Read the model definition and answer for the solid it produces. Units are mm, in the model's axes. Face numbers are marked on the shaded views. Give positions to 0.01 mm unless a question says otherwise; leave off trailing zeros. Write each loop counter-clockwise with the first axis right and the second up, starting at its lowest first coordinate (ties: lowest second). Pieces come first, ordered by that corner, then holes. Notation, with made-up numbers: M 21,-32 L 66,-32 A12 ccw 66,-22 Z; hole C 65,-18 d10. An arc over 180 degrees is marked long. Write each question's results on one line, items separated by ' | '. Start each with the question number.
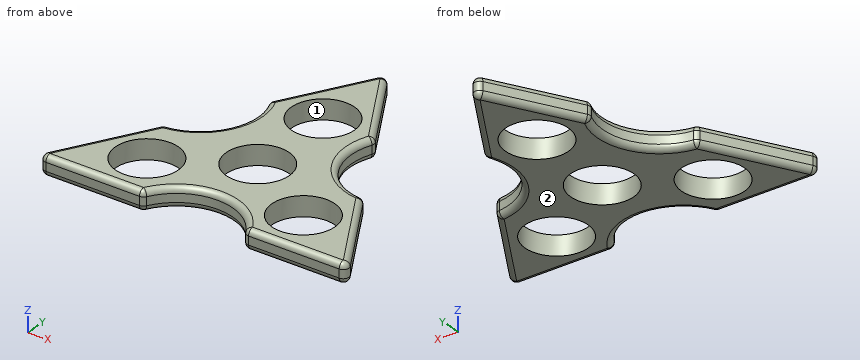
```python
from build123d import *

# Parameters (mm, degrees)
F0_R     = 11.15
F1_DEPTH = 7
F2_R     = 2


# Not quite as in the source:
# - a feature names something its author has since deleted; it is built from what else it names


with BuildPart() as f1:
    # F0 (on Top) → F1 (new body)
    with BuildSketch(Plane.XY):
        with BuildLine():
            Line((18.6057756776, 31.4331508418), (0, 63.6592996296))
            Line((0, 63.6592996296), (-18.6057756776, 31.4331508418))
            ThreePointArc((-18.6057756776, 31.4331508418), (-19.2524106529, 12.6478352194), (-35.1976537124, 2.6951750926))
            Line((-35.1976537124, 2.6951750926), (-55.1305706664, -31.8296498148))
            Line((-55.1305706664, -31.8296498148), (-17.4760334194, -31.8296498148))
            ThreePointArc((-17.4760334194, -31.8296498148), (0.5244189685, -20.546513576), (18.5248713564, -31.8296498148))
            Line((18.5248713564, -31.8296498148), (55.1305706664, -31.8296498148))
            Line((55.1305706664, -31.8296498148), (35.1976537124, 2.6951750926))
            ThreePointArc((35.1976537124, 2.6951750926), (19.2524106529, 12.6478352194), (18.6057756776, 31.4331508418))
        make_face()
        with Locations((-27.5652853332, -15.9148249074)):
            Circle(F0_R, mode=Mode.SUBTRACT)
        with Locations((27.5652853332, -15.9148249074)):
            Circle(F0_R, mode=Mode.SUBTRACT)
        Circle(F0_R, mode=Mode.SUBTRACT)
        with Locations((0, 31.8296498148)):
            Circle(F0_R, mode=Mode.SUBTRACT)
    extrude(amount=F1_DEPTH)

    # F2
    f2_edges = [f1.edges().sort_by_distance(p)[0] for p in [
        (55.130571, -31.82965, 3.5),
        (35.197654, 2.695175, 3.5),
        (45.164112, -14.567237, 0),
        (45.164112, -14.567237, 7),
        (18.605776, 31.433151, 3.5),
        (19.252411, 12.647835, 0),
        (19.252411, 12.647835, 7),
        (0, 63.6593, 3.5),
        (9.302888, 47.546225, 0),
        (9.302888, 47.546225, 7),
        (-18.605776, 31.433151, 3.5),
        (-9.302888, 47.546225, 0),
        (-9.302888, 47.546225, 7),
        (-35.197654, 2.695175, 3.5),
        (-19.252411, 12.647835, 0),
        (-19.252411, 12.647835, 7),
        (-55.130571, -31.82965, 3.5),
        (-45.164112, -14.567237, 0),
        (-45.164112, -14.567237, 7),
        (-17.476033, -31.82965, 3.5),
        (18.524871, -31.82965, 3.5),
        (0.524419, -20.546514, 0),
        (0.524419, -20.546514, 7),
        (-36.303302, -31.82965, 0),
        (-36.303302, -31.82965, 7),
        (36.827721, -31.82965, 0),
        (36.827721, -31.82965, 7),
    ]]
    fillet(f2_edges, radius=F2_R)


solid = f1.part
```
Item 1: Straight lines are drawn through the part: line 1 (Y direction, x = 0, z = 3); line 2 (Y direction, x = 0, z = 5.25); line 3 (X direction, y = -16, z = 1.75). For each, find the intervals that lie inside material, in ascending order.
Item 2: Section A-A, the plane z = 3.75 is taken. Determine the outline of the cut face in (x, y).
Item 3: Given P1, Ø1, axis at x = 29.5, z = 2, coming from the +Y side; P2, Ø3, axis at x = 41, z = 2, coming from the +Y side; P3, Ø1, axis at x = 24.5, z = 2, coming from the +Y side, each flat-ended and moving along its own axis, determine where each tip first touches the part or whether it passes through.
Item 4: Determine the mould class of the marked faces 1 and 2 for opening direction Y: +Y half, -Y half, draft (parallel to the pull), parting line (faces both ways), or undercut.
Worked out:
1) line 1: y = -20.55 to -11.15, 11.15 to 20.68, 42.98 to 61.66 | line 2: y = -20.54 to -11.15, 11.15 to 20.68, 42.98 to 61.64 | line 3: x = -45.97 to -38.71, -16.42 to 16.42, 38.71 to 45.97
2) outline: M -53.4,-28.83 A2 ccw -51.67,-31.83 L -18.69,-31.83 A2 ccw -16.94,-30.8 A20 cw 17.99,-30.8 A2 ccw 19.74,-31.83 L 51.67,-31.83 A2 ccw 53.4,-28.83 L 35.71,1.8 A2 ccw 34.22,2.79 A20 cw 18.2,30.54 A2 ccw 18.09,32.33 L 1.73,60.66 A2 ccw -1.73,60.66 L -18.09,32.33 A2 ccw -18.2,30.54 A20 cw -34.22,2.79 A2 ccw -35.71,1.8 Z; hole C -27.57,-15.91 d22.3; hole C 0,0 d22.3; hole C 0,31.83 d22.3; hole C 27.57,-15.91 d22.3
3) P1: stops at y = 4.14 | P2: stops at y = -4.76 | P3: stops at y = 7.09
4) face 1: undercut | face 2: draft
